Read the model definition and answer for the solid it produces. Units are mm, in the model's axes. A direction names the side the tool comes from. Give positions to 0.01 mm unless a question says otherwise; leave off trailing zeros. Loops run counter-clockwise (first coordinate to the right, second up) from the corner with the lowest first, then second, coordinate; pieces in that order, holes last. Notation, with made-up numbers: (42.5, 13.5) - (68.5, 13.5) arc R7 ccw to (68.5, 24.5) - close; hole circle Ø8 at (72.5, 34.5). An arc over 180 degrees is marked (long way). Write item = value, one per line.
```python
from build123d import *

# Parameters (mm, degrees)
SKETCH_1_W          = 30
SKETCH_1_H          = 50
SKETCH_1_R          = 1.6
EXTRUDE_1_DEPTH     = 3
SKETCH_2_W          = 5
SKETCH_2_H          = 36
EXTRUDE_2_DEPTH     = 8
SKETCH_5_R          = 1.6
CUT_EXTRUDE_1_DEPTH = 10
SKETCH_6_W          = 5
SKETCH_6_H          = 7
EXTRUDE_3_DEPTH     = 30
RIB_1_REACH         = 65.828
SKETCH_7_WALL_W     = 168.57168005
SKETCH_7_WALL_H     = 7


with BuildPart() as part:
    # 草图1 → 凸台-拉伸1 (new body)
    with BuildSketch(Plane.XY):
        with Locations((-25, -15)):
            Rectangle(SKETCH_1_W, SKETCH_1_H)
        with Locations((-14, 5.5)):
            Circle(SKETCH_1_R, mode=Mode.SUBTRACT)
        with Locations((-36, -35.5)):
            Circle(SKETCH_1_R, mode=Mode.SUBTRACT)
        with Locations((-14, -35.5)):
            Circle(SKETCH_1_R, mode=Mode.SUBTRACT)
        with Locations((-36, 5.5)):
            Circle(SKETCH_1_R, mode=Mode.SUBTRACT)
    extrude(amount=EXTRUDE_1_DEPTH)

    # 草图2 → 凸台-拉伸2 (add)
    with BuildSketch(Plane.XY.offset(3)):
        with Locations((-20.894219559, -15)):
            Rectangle(SKETCH_2_W, SKETCH_2_H)
    extrude(amount=EXTRUDE_2_DEPTH)

    # 草图5 → 切除-拉伸1 (cut)
    with BuildSketch(Plane(origin=(-18.394219559, 0, 0), x_dir=(0, 0, -1), z_dir=(1, 0, 0))):
        with Locations(Location((-7, -0.268, 0), (0, 0, 90))):
            Circle(SKETCH_5_R)
        with Locations(Location((-7, -29.732, 0), (0, 0, 90))):
            Circle(SKETCH_5_R)
    extrude(amount=-CUT_EXTRUDE_1_DEPTH, mode=Mode.SUBTRACT)

    # 草图6 → 凸台-拉伸3 (add)
    with BuildSketch(Plane.XY.offset(11)):
        with Locations((-20.894219559, -15.339980262)):
            Rectangle(SKETCH_6_W, SKETCH_6_H)
    extrude(amount=EXTRUDE_3_DEPTH)

    # 草图7 wall → 筋1 (add, up to next)
    with BuildSketch(Plane(origin=(-14.197109779, -11.839980262, 22), x_dir=(0.215700425519, 0, -0.97645958771), z_dir=(-0.97645958771, 0, -0.215700425519)), mode=Mode.PRIVATE) as rib_1_sk1:
        with Locations((0, 3.5)):
            Rectangle(SKETCH_7_WALL_W, SKETCH_7_WALL_H)
    rib_1_tool1 = extrude(rib_1_sk1.sketch, amount=RIB_1_REACH, mode=Mode.PRIVATE) - part.part
    add(rib_1_tool1.solids().sort_by_distance((-14.197109779, -11.839980262, 22))[0])


solid = part.part
```
1) A cutting plane is placed at D-D on x = -36. Determine the outline of the cut face in (y, z), then the cut area to 3 significant figures.
Output:
outline = (-40, 0) - (-37.1, 0) - (-37.1, 3) - (-40, 3) - close; (-33.9, 0) - (3.9, 0) - (3.9, 3) - (-33.9, 3) - close; (7.1, 0) - (10, 0) - (10, 3) - (7.1, 3) - close
area = 131 mm²
2) A cutting plane is placed at C-C on z = 7. Determine the outline of the cut face in (x, y).
Output:
outline = (-23.39, -33) - (-18.39, -33) - (-18.39, -31.33) - (-23.39, -31.33) - close; (-23.39, -28.13) - (-18.39, -28.13) - (-18.39, -18.84) - (-10.88, -18.84) - (-10.88, -11.84) - (-18.39, -11.84) - (-18.39, -1.87) - (-23.39, -1.87) - close; (-23.39, 1.33) - (-18.39, 1.33) - (-18.39, 3) - (-23.39, 3) - close
3) A cutting plane is placed at A-A on x = -22. Determine the outline of the cut face in (y, z).
Output:
outline = (-40, 0) - (10, 0) - (10, 3) - (3, 3) - (3, 11) - (-11.84, 11) - (-11.84, 41) - (-18.84, 41) - (-18.84, 11) - (-33, 11) - (-33, 3) - (-40, 3) - close; hole circle Ø3.2 at (-29.73, 7); hole circle Ø3.2 at (-0.27, 7)
4) A tool of negligible diameter and unlimited length cuts with its end or side. For faces 1 (the face through (-21, -4, 11)), 2 (the face through (-21, -33, 7)), 3 (the face through (-18.394, -26, 7)), 4 (the face through (-18.394, -5, 7)), 5 (the face through (-15.27, -36.47, 1.48)), from which of +Z, -Z, +X, -X, +Y, -Y can it reach the whole face along a straight path? Write none if from no direction.
Output:
face_1 = +Z, +X, -X, +Y
face_2 = +Z, +X, -X, -Y
face_3 = +Z, +X, -Y
face_4 = +Z, +X, +Y
face_5 = +Z, -Z
5) Each of these flat-tipped pins is pushed along its axis until it touches: P1, Ø2, axis at x = -16.5, z = 11.5, coming from the -Y side; P2, Ø6.5, axis at y = -25.5, z = 6.5, coming from the +X side; P3, Ø6.5, axis at x = -15.5, z = 13, coming from the +Y side. Where does it stop, or does it pass through?
Output:
P1 = -18.84
P2 = -18.39
P3 = -11.84
6) A cutting plane is placed at B-B on y = 5.5. Determine the outline of the cut face in (x, z).
Output:
outline = (-40, 0) - (-37.6, 0) - (-37.6, 3) - (-40, 3) - close; (-34.4, 0) - (-15.6, 0) - (-15.6, 3) - (-34.4, 3) - close; (-12.4, 0) - (-10, 0) - (-10, 3) - (-12.4, 3) - close
7) Find the intervals of material crossed by probe 1 along Y at (x, z) = (-36, 1); probe 2 along X at (y, z) = (-35, 2); probe 3 along Z at (x, y) = (-21, -36.5), in increasing order.
Output:
probe_1 = -40 to -37.1, -33.9 to 3.9, 7.1 to 10
probe_2 = -40 to -37.52, -34.48 to -15.52, -12.48 to -10
probe_3 = 0 to 3
8) The mould has two halves that part along X. Classify faces 6 (the face through (-19, -18.84, 22)), 7 (the face through (-40, -15, 1)), 8 (the face through (-35.26, -36.92, 1.48)): pulls with the +X half, pulls with the -X half, needs draft (parallel to the pull), parting line crosses it, or undercut.
Output:
face_6 = needs draft
face_7 = pulls with the -X half
face_8 = undercut
